from build123d import *

# Parameters (mm, degrees)
F0_W      = 133.096
F0_H      = 50.8
F1_DEPTH  = 12.7
F2_W      = 56.896
F2_H      = 50.8
F3_DEPTH  = 56.896
F4_SIZE2  = 53.848
F4_SIZE   = 19.6088
F5_R      = 14.2875
F6_DEPTH  = 50.8
F7_R      = 28.44799
F9_R      = 7.874
F8_R      = 7.874
F10_DEPTH = 25.4


# Not quite as in the source:
# - a fillet or chamfer is up to 0.001 mm smaller than in the source, because OpenCascade refuses the exact size


with BuildPart() as f1:
    # F0 (on Top) → F1 (new body)
    with BuildSketch(Plane.XY):
        with Locations((66.548, -25.4)):
            Rectangle(F0_W, F0_H)
    extrude(amount=F1_DEPTH)

    # F2 (on face) → F3 (join)
    with BuildSketch(Plane.XY.offset(12.7)):
        with Locations((66.548, -25.4)):
            Rectangle(F2_W, F2_H)
    extrude(amount=F3_DEPTH)

    # F4
    f4_edges = [f1.edges().sort_by_distance(p)[0] for p in [
        (66.548, -50.8, 69.596),
    ]]
    f4_side = f1.faces().sort_by_distance((66.548, -25.4, 69.596))[0]
    chamfer(f4_edges, length=F4_SIZE, length2=F4_SIZE2, reference=f4_side)

    # F5 (on face) → F6 (cut)
    with BuildSketch(Plane(origin=(0, 0, 0), x_dir=(-1, 0, 0), z_dir=(0, 1, 0))):
        with Locations((-66.548, 41.148)):
            Circle(F5_R)
    extrude(amount=-F6_DEPTH, mode=Mode.SUBTRACT)

    # F7 (radius 28.448 in the source; OpenCascade refuses exactly that, so slightly less here)
    f7_edges = [f1.edges().sort_by_distance(p)[0] for p in [
        (94.996, -15.5956, 69.596),
        (38.1, -15.5956, 69.596),
    ]]
    fillet(f7_edges, radius=F7_R)

    # F9 (on face) + F8 (on face) → F10 (cut)
    with BuildSketch(Plane(origin=(0, 0, 0), x_dir=(1, 0, 0), z_dir=(0, 0, -1))):
        with Locations((18.796, 25.4)):
            Circle(F9_R)
    with BuildSketch(Plane(origin=(0, 0, 0), x_dir=(1, 0, 0), z_dir=(0, 0, -1))):
        with Locations((114.3, 25.4)):
            Circle(F8_R)
    extrude(amount=-F10_DEPTH, mode=Mode.SUBTRACT)


solid = f1.part
Design review of the part built by this model. Coordinates are the model's own, in mm. A direction names the side the tool comes from. Give positions to 0.01 mm unless a question says otherwise; leave off trailing zeros. Loops run counter-clockwise (first coordinate to the right, second up) from the corner with the lowest first, then second, coordinate; pieces in that order, holes last. Notation, with made-up numbers: (37, -27.75) -> (79, -27.75) arc R15 cw to (79, -18.75) -> close; hole circle Ø3 at (46.25, 52.25). An arc over 180 degrees is marked (long way). One line per question, with ' | ' between items. Start each with the question number.
(1) Insertion check: P1, Ø3, axis at x = 60.5, y = -11.5, coming from the -Z side; P2, Ø3, axis at y = -8, z = 45, coming from the +X side; P3, Ø23, axis at y = -17.5, z = 30.5, coming from the +X side; P4, Ø18, axis at x = 114.3, y = -25.4, coming from the +Z side. Each pin has a flat end and moves straight along its axis. Give the tip position at first contact, or say it passes through.
(2) We need section B-B (y = -25.4). State how many separate pieces and enclosed holes the cut face has, and give its area (3 significant figures).
(3) We need section D-D (x = 97). State the section outline as (y, z) points, and give its area (3 significant figures).
(4) For faces 1 (the face through (38.1, -26, 27)), 2 (the face through (94.996, -26, 27)), 3 (the face through (66, -50.8, 6)), list the 3-axis set-ups (+Z, -Z, +X, -X, +Y, -Y) from which the entire face can be reached by the end or side of a thin tool; tool diameter is ignored.
(5) Draft analysis for pull direction Y (two halves, no side actions). For faces 4 (the face through (105, -25, 12.7)), 5 (the face through (10.93, -25.75, 6.26)), 6 (the face through (65.6, 0, 26.6)), state which applies: +Y half, -Y half, draft (parallel to the pull), parting line (faces both ways), or undercut.
(6) For line 1 (X direction, y = -25.4, z = 9); line 2 (Y direction, x = 114.3, z = 8.75); line 3 (X direction, y = -20, z = 48), list the stretches that pass through material, from the lowest coordinate up.
(7) We need section A-A (x = 114.3). State the section outline as (y, z) points.
The answers:
1) P1: stops at z = 0 | P2: stops at x = 94.9 | P3: stops at x = 95 | P4: stops at z = 12.7
2) separate pieces: 3 | enclosed holes: 1 | area: 3,540 mm^2
3) outline: (-50.8, 0) -> (0, 0) -> (0, 12.7) -> (-50.8, 12.7) -> close | area: 645 mm^2
4) face 1: +Z, -X, +Y, -Y | face 2: +Z, +X, +Y, -Y | face 3: +Z, -Z, +X, -X, -Y
5) face 4: draft | face 5: undercut | face 6: +Y half
6) line 1: x = 0 to 10.92, 26.67 to 106.43, 122.17 to 133.1 | line 2: y = -50.8 to -33.27, -17.53 to 0 | line 3: x = 38.94 to 54.01, 79.09 to 94.16
7) outline: (-50.8, 0) -> (-33.27, 0) -> (-33.27, 12.7) -> (-50.8, 12.7) -> close; (-17.53, 0) -> (0, 0) -> (0, 12.7) -> (-17.53, 12.7) -> close
